```python
from build123d import *

# Parameters (mm, degrees)
SKETCH_1_R      = 6
EXTRUDE_1_DEPTH = 1
SKETCH_2_R      = 5
SKETCH_2_R_2    = 3.9
EXTRUDE_2_DEPTH = 8
CHAMFER_1_SIZE  = 1
CHAMFER_2_SIZE  = 1


with BuildPart() as part:
    # Эскиз1 → Бобышка-Вытянуть1 (new body)
    with BuildSketch(Plane(origin=(0, 0, 0), x_dir=(1, 0, 0), z_dir=(0, 1, 0))):
        with Locations(Location((0, 0, 0), (0, 0, 270))):
            Circle(SKETCH_1_R)
    extrude(amount=EXTRUDE_1_DEPTH)

    # Эскиз2 → Бобышка-Вытянуть2 (add)
    with BuildSketch(Plane(origin=(0, 1, 0), x_dir=(1, 0, 0), z_dir=(0, 1, 0))):
        with Locations(Location((0, 0, 0), (0, 0, 270))):
            Circle(SKETCH_2_R)
        with Locations(Location((0, 0, 0), (0, 0, 270))):
            Circle(SKETCH_2_R_2, mode=Mode.SUBTRACT)
    extrude(amount=EXTRUDE_2_DEPTH)

    # Фаска1
    chamfer_1_edges = [part.edges().sort_by_distance(p)[0] for p in [
        (0, 1, -6),
    ]]
    chamfer(chamfer_1_edges, length=CHAMFER_1_SIZE - 0.0001)  # a hair under: the kernel refuses the full size

    # Фаска2
    chamfer_2_edges = [part.edges().sort_by_distance(p)[0] for p in [
        (0, 9, -5),
    ]]
    chamfer(chamfer_2_edges, length=CHAMFER_2_SIZE)


solid = part.part
```
Verification items for the finished model (mm, model axes). Give positions to 0.01 mm unless a question says otherwise; leave off trailing zeros. Loops run counter-clockwise (first coordinate to the right, second up) from the corner with the lowest first, then second, coordinate; pieces in that order, holes last.
1. Section check C-C, the plane y = 1.5. Enter the section's corners in (x, z), then the cut area to 3 significant figures.
2. Go/stop test with flat-tipped pins: pin 1 Ø5 at (y, z) = (5, -3) entering from -X; pin 2 Ø4 at (y, z) = (4, 4.5) entering from +X; pin 3 Ø1 at (y, z) = (4.5, -0.5) entering from +X. Record where each tip stops, or that it passes through.
3. Thickness scan on line 1 (X direction, y = 3.75, z = 0); line 2 (X direction, y = 3.5, z = 3.25); line 3 (Y direction, x = 0.25, z = 3.75). Record the ranges inside material, lowest first.
4. Mould release check, pull along Z, two halves, no side actions. Record for faces 1 (the flat face through (0, 0, 0)), 2 (the cylindrical face through (-4.88, 4.45, -1.08)), 3 (the cylindrical face through (-2.373, 4.944, -3.095)): released by +Z, released by -Z, zero draft, split by the parting line, or undercut.
Geometry says:
1. outline: circle Ø10 at (0, 0); hole circle Ø7.8 at (0, 0)
1. area: 30.8 mm2
2. pin 1: stops at x = -4.97
2. pin 2: stops at x = 4.33
2. pin 3: stops at x = 5
3. line 1: x = -5 to -3.9, 3.9 to 5
3. line 2: x = -3.8 to -2.16, 2.16 to 3.8
3. line 3: y = 0 to 1
4. face 1: zero draft
4. face 2: split by the parting line
4. face 3: undercut
